Input: part model. Units: mm. Frame: model coordinates. A direction names the side the tool comes from. Give positions to 0.01 mm unless a question says otherwise; leave off trailing zeros. Loops run counter-clockwise (first coordinate to the right, second up) from the corner with the lowest first, then second, coordinate; pieces in that order, holes last. Notation, with made-up numbers: (53.25, 72) -> (63.25, 72) arc R12 cw to (63.25, 92) -> close; hole circle Ø2 at (77.5, 24.25). An arc over 180 degrees is marked (long way). Answer as a JSON object with one key per item and string values.
```python
from build123d import *

# Parameters (mm, degrees)
SALIENTE_EXTRUIR1_DEPTH = 15
CORTAR_EXTRUIR1_DEPTH   = 477.91260816
REDONDEO1_R             = 220
REDONDEO2_R             = 70
REDONDEO3_R             = 15
REDONDEO4_R             = 30
CROQUIS7_R              = 14.29
CORTAR_EXTRUIR5_DEPTH   = 477.91260816
CROQUIS8_R              = 14.29
CORTAR_EXTRUIR6_DEPTH   = 523
CROQUIS9_R              = 14.289999998
CORTAR_EXTRUIR7_DEPTH   = 10
CROQUIS12_R             = 12.5
CORTAR_EXTRUIR10_DEPTH  = 10
CROQUIS13_R             = 2.02
CORTAR_EXTRUIR11_DEPTH  = 10
CORTAR_EXTRUIR12_DEPTH  = 477.91260816
REDONDEO5_R             = 40
CORTAR_EXTRUIR13_DEPTH  = 429.858749969
REDONDEO6_R             = 40


with BuildPart() as part:
    # Croquis1 → Saliente-Extruir1 (new body)
    with BuildSketch(Plane(origin=(0, 0, 0), x_dir=(0, 0, -1), z_dir=(1, 0, 0))):
        with BuildLine():
            Line((65, 25.4), (65, 281.06162282))
            Line((65, 281.06162282), (385, 281.06162282))
            Line((385, 281.06162282), (385, -8.93837718))
            Line((385, -8.93837718), (205, -8.93837718))
            Line((205, -8.93837718), (205, 22.4))
            Line((205, 22.4), (115, 22.4))
            Line((115, 22.4), (114.819347292, 22.4))
            ThreePointArc((114.819347292, 22.4), (88.497282844, 0.445204045), (65, 25.4))
        make_face()
    extrude(amount=SALIENTE_EXTRUIR1_DEPTH)

    # Croquis2 → Cortar-Extruir1 (cut, through all)
    with BuildSketch(Plane.ZY):
        Polygon((-82.667651581, 25.4), (-86.333825791, 31.75), (-93.666174209, 31.75), (-97.332348419, 25.4), (-93.666174209, 19.05), (-86.333825791, 19.05), align=None)
    extrude(amount=-CORTAR_EXTRUIR1_DEPTH, mode=Mode.SUBTRACT)

    # Redondeo1
    redondeo1_edges = [part.edges().sort_by_distance(p)[0] for p in [
        (7.5, 281.06162282, -385),
    ]]
    fillet(redondeo1_edges, radius=REDONDEO1_R)

    # Redondeo2
    redondeo2_edges = [part.edges().sort_by_distance(p)[0] for p in [
        (7.5, 281.06162282, -65),
    ]]
    fillet(redondeo2_edges, radius=REDONDEO2_R)

    # Redondeo3
    redondeo3_edges = [part.edges().sort_by_distance(p)[0] for p in [
        (7.5, -8.93837718, -205),
        (7.5, 22.4, -205),
    ]]
    fillet(redondeo3_edges, radius=REDONDEO3_R)

    # Redondeo4
    redondeo4_edges = [part.edges().sort_by_distance(p)[0] for p in [
        (7.5, -8.93837718, -385),
    ]]
    fillet(redondeo4_edges, radius=REDONDEO4_R)

    # Croquis7 → Cortar-Extruir5 (cut, through all)
    with BuildSketch(Plane(origin=(15, 0, 0), x_dir=(0, 0, -1), z_dir=(1, 0, 0))):
        with Locations((354.499999998, 21.561622823)):
            Circle(CROQUIS7_R)
    extrude(amount=-CORTAR_EXTRUIR5_DEPTH, mode=Mode.SUBTRACT)

    # Croquis8 → Cortar-Extruir6 (cut)
    with BuildSketch(Plane(origin=(15, 0, 0), x_dir=(0, 0, -1), z_dir=(1, 0, 0))):
        with Locations((299.999999998, 151.061622823)):
            Circle(CROQUIS8_R)
    extrude(amount=-CORTAR_EXTRUIR6_DEPTH, mode=Mode.SUBTRACT)

    # Croquis9 → Cortar-Extruir7 (cut)
    with BuildSketch(Plane(origin=(15, 0, 0), x_dir=(0, 0, -1), z_dir=(1, 0, 0))):
        with Locations((184.499999998, 231.061622823)):
            Circle(CROQUIS9_R)
    extrude(amount=-CORTAR_EXTRUIR7_DEPTH, mode=Mode.SUBTRACT)

    # Croquis12 → Cortar-Extruir10 (cut)
    with BuildSketch(Plane.ZY):
        with Locations((-267.424734061, 207.135375692)):
            Circle(CROQUIS12_R)
    extrude(amount=-CORTAR_EXTRUIR10_DEPTH, mode=Mode.SUBTRACT)

    # Croquis13 → Cortar-Extruir11 (cut)
    with BuildSketch(Plane.ZY):
        with Locations((-263.175315265, 232.177389187)):
            Circle(CROQUIS13_R)
        with Locations((-271.674152858, 182.093362197)):
            Circle(CROQUIS13_R)
    extrude(amount=-CORTAR_EXTRUIR11_DEPTH, mode=Mode.SUBTRACT)

    # Croquis14 → Cortar-Extruir12 (cut, through all)
    with BuildSketch(Plane(origin=(15, 0, 0), x_dir=(0, 0, -1), z_dir=(1, 0, 0))):
        with BuildLine():
            Line((65, 72.4), (270, 72.4))
            ThreePointArc((270, 72.4), (274.363902477, 93.8541681), (271.886825139, 115.607077366))
            ThreePointArc((271.886825139, 115.607077366), (293.695729554, 182.870527235), (360.959179423, 161.06162282))
            Line((360.959179423, 161.06162282), (409.037931036, 257.33581614))
            Line((409.037931036, 257.33581614), (105.335360325, 302.08857435))
            Line((105.335360325, 302.08857435), (0, 212.58305793))
            Line((0, 212.58305793), (65, 72.4))
        make_face()
    extrude(amount=-CORTAR_EXTRUIR12_DEPTH, mode=Mode.SUBTRACT)

    # Redondeo5
    # the kernel refuses this fillet: 40 mm, written as the material it adds along each edge
    with BuildSketch(Plane(origin=(15, 72.4, -270), x_dir=(0, 0.9990478553757552, -0.04362777405625806), z_dir=(-1, 0, 0))) as redondeo5_piece_1:
        with BuildLine():
            CenterArc((38.304739361, -39.69334508), REDONDEO5_R, 82.900783035, 94.598735985)
            Line((-1.657174854, -37.948234118), (0, 0))
            ThreePointArc((0, 0), (21.62412798, 3.423749812), (43.24825596, 0))
        make_face()
    extrude(amount=15)
    # the kernel refuses this fillet: 40 mm, written as the material it takes off along each edge
    with BuildSketch(Plane(origin=(115, 72.4, -65), x_dir=(0, 0, -1), z_dir=(-1, 0, 0))) as redondeo5_2_piece_1:
        with BuildLine():
            CenterArc((REDONDEO5_R, REDONDEO5_R), REDONDEO5_R, 180, 90)
            Line((0, REDONDEO5_R), (0, 0))
            Line((0, 0), (REDONDEO5_R, 0))
        make_face()
    extrude(amount=215, mode=Mode.SUBTRACT)

    # Croquis15 → Cortar-Extruir13 (cut, through all)
    with BuildSketch(Plane(origin=(15, 0, 0), x_dir=(0, 0, -1), z_dir=(1, 0, 0))):
        with BuildLine():
            Line((316.423002092, 188.334350093), (358.626196651, 190.922485321))
            Line((358.626196651, 190.922485321), (422.761195779, 101.204099428))
            Line((422.761195779, 101.204099428), (385, 21.06162282))
            ThreePointArc((385, 21.06162282), (371.881027209, 113.376882144), (316.423002092, 188.334350093))
        make_face()
    extrude(amount=-CORTAR_EXTRUIR13_DEPTH, mode=Mode.SUBTRACT)

    # Redondeo6
    # the kernel refuses this fillet: 40 mm, written as the material it takes off along each edge
    with BuildSketch(Plane(origin=(154.505258907, 188.334350093, -316.423002092), x_dir=(0, -0.5580210387586911, 0.8298268013885014), z_dir=(-1, 0, 0))) as redondeo6_piece_1:
        with BuildLine():
            CenterArc((33.481262138, -33.19307214), REDONDEO6_R, 56.080950645, 115.615192881)
            ThreePointArc((-6.099380681, -27.416159986), (-3.556977801, -13.595221761), (0, 0))
            ThreePointArc((0, 0), (27.901051781, 8.508659825), (55.802103563, 0))
        make_face()
    extrude(amount=294.010517815, mode=Mode.SUBTRACT)


solid = part.part
```
Q1. Draft query along Z for faces 1 (the cylindrical face through (7.605, 181.393, -299.639)), 2 (the cylindrical face through (7.6, 18.12, -200.49)), 3 (the flat face through (7, 29, -65)). Return one class per face: +Z half, -Z half, draft (parallel to the pull), parting line (faces both ways), or undercut.
Evaluation:
{"face 1": "parting line", "face 2": "undercut", "face 3": "+Z half"}
Q2. Access query for faces 4 (the cylindrical face through (7.6, -4.66, -209.51)), 5 (the flat face through (0, 66, -265)), 6 (the flat face through (8, 72.4, -168)), 7 (the flat face through (7, 19.05, -90)). Directions: +Z, -Z, +X, -X, +Y, -Y. A direction counts if a zero-diameter tool reaches every point of the face in a straight line with its end or side. Return the directions, or none.
Evaluation:
{"face 4": "+X, -X, -Y", "face 5": "+Z, -Z, -X, +Y, -Y", "face 6": "+Z, +X, -X, +Y", "face 7": "+X, -X"}
Q3. Section B-B, the plane x = 5.5. Return the cut outline in (y, z).
Evaluation:
{"outline": "(-8.94, -355) arc R30 ccw to (21.06, -385) -> (61.06, -385) arc R220 ccw to (61.55, -385) arc R190 ccw to (168.99, -336.78) arc R40 ccw to (157.2, -270.12) arc R50 ccw to (115.61, -271.89) arc R40 cw to (72.4, -232.02) -> (72.4, -105) arc R40 ccw to (32.4, -65) -> (25.4, -65) arc R25 ccw to (22.4, -114.82) -> (22.4, -190) arc R15 cw to (7.4, -205) -> (6.06, -205) arc R15 ccw to (-8.94, -220) -> close; hole circle Ø28.58 at (21.56, -354.5); hole (19.05, -93.67) -> (25.4, -97.33) -> (31.75, -93.67) -> (31.75, -86.33) -> (25.4, -82.67) -> (19.05, -86.33) -> close; hole circle Ø28.58 at (151.06, -300)"}
Q4. Ray query, line 1 along Z through (x, y) = (7, 26.5); line 2 along Y through (x, z) = (9.25, -135.5); line 3 along Y through (x, z) = (11.5, -300). Return the intervals inside material, ascending.
Evaluation:
{"line 1": "z = -385 to -367.91, -341.09 to -96.7, -83.3 to -65", "line 2": "y = 22.4 to 72.4", "line 3": "y = -8.94 to 136.77, 165.35 to 181.46"}
Q5. Section D-D, the plane z = -177. Return the cut outline in (x, y).
Evaluation:
{"outline": "(0, 22.4) -> (15, 22.4) -> (15, 72.4) -> (0, 72.4) -> close"}
Q6. Pin query (flat end, axial travel): pin 1 (6 mm diameter, centred on x = 7.5, z = -89.5, fed in from +Y); pin 2 (8 mm diameter, centred on x = 11, z = -89, fed in from -Y); pin 3 (1.1 mm diameter, centred on x = 6, y = 7, fed in from +Z); pin 4 (1 mm diameter, centred on y = 44, z = -247, fed in from -X). Return the tip coordinate at first contact, or that it passes through.
Evaluation:
{"pin 1": "stops at y = 70.4", "pin 2": "stops at y = 0.4", "pin 3": "stops at z = -72.5", "pin 4": "stops at x = 0"}
Q7. Section A-A, the plane z = -90. Return the cut outline in (x, y).
Evaluation:
{"outline": "(0, 0.4) -> (15, 0.4) -> (15, 19.05) -> (0, 19.05) -> close; (0, 31.75) -> (15, 31.75) -> (15, 69.48) -> (0, 69.48) -> close"}
Q8. Section C-C, the plane z = -311. Return the cut outline in (x, y).
Evaluation:
{"outline": "(0, -8.94) -> (15, -8.94) -> (15, 141.94) -> (0, 141.94) -> close; (0, 160.18) -> (15, 160.18) -> (15, 181.92) -> (0, 181.92) -> close"}
